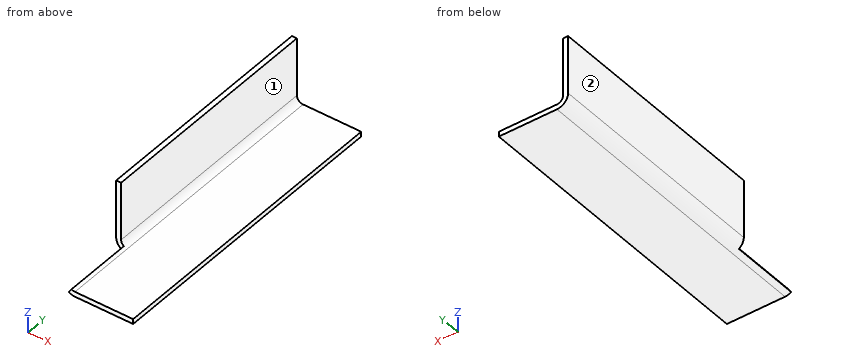
from build123d import *

# Parameters (mm, degrees)
SKETCH1_W                    = 28
SKETCH1_H                    = 122
BASE_FLANGE1_DEPTH           = 2
EDGE_FLANGE1_STRIP_W         = 13
EDGE_FLANGE1_STRIP_H         = 2
EDGE_FLANGE1_STRIP_CUT_DEPTH = 122
EDGE_FLANGE1_DEPTH           = 122
CUT_EXTRUDE1_START           = -61
CUT_EXTRUDE1_DEPTH           = 28


# Read off the part's stored shape, not the designer's step: Cut-Extrude1
# Sheet-metal steps are written as plain solids
with BuildPart() as part:
    # Sketch1 → Base-Flange1 (new body)
    with BuildSketch(Plane(origin=(0, 0, 0), x_dir=(0, 0, -1), z_dir=(1, 0, 0))):
        Rectangle(SKETCH1_W, SKETCH1_H)
    extrude(amount=-BASE_FLANGE1_DEPTH)

    # Edge-Flange1 strip (across the edge) → Edge-Flange1 strip cut (cut)
    with BuildSketch(Plane(origin=(0, -61, -14), x_dir=(0, 0, 1), z_dir=(0, 1, 0))):
        with Locations((-2, -1)):
            Rectangle(EDGE_FLANGE1_STRIP_W, EDGE_FLANGE1_STRIP_H)
    extrude(amount=EDGE_FLANGE1_STRIP_CUT_DEPTH, mode=Mode.SUBTRACT)

    # Edge-Flange1 section (across the edge) → Edge-Flange1 (add)
    with BuildSketch(Plane(origin=(0, -61, -14), x_dir=(0, 0, 1), z_dir=(0, 1, 0))):
        with BuildLine():
            Line((0, 2.5), (0, 26))
            Line((0, 26), (2, 26))
            Line((2, 26), (2, 2.5))
            ThreePointArc((2, 2.5), (2.732233047, 0.732233047), (4.5, 0))
            Line((4.5, 0), (4.5, -2))
            ThreePointArc((4.5, -2), (1.318019485, -0.681980515), (0, 2.5))
        make_face()
    extrude(amount=EDGE_FLANGE1_DEPTH)

    # Cut-Extrude1 outline → Cut-Extrude1 (cut)
    with BuildSketch(Plane(origin=(0, 0, 0), x_dir=(1, 0, 0), z_dir=(0, 1, 0)).offset(CUT_EXTRUDE1_START)):
        with BuildLine():
            Line((1.111111111, 11.578698548), (0, 13.241657386))
            ThreePointArc((0, 13.241657386), (-1.468626966, 11.621320343), (-2, 9.5))
            Line((-2, 9.5), (-2, -14))
            Line((-2, -14), (0, -14))
            Line((0, -14), (0, 9.5))
            ThreePointArc((0, 9.5), (0.295207241, 10.678511302), (1.111111111, 11.578698548))
        make_face()
    extrude(amount=CUT_EXTRUDE1_DEPTH, mode=Mode.SUBTRACT)


solid = part.part
Check sheet for the modelled part. Datum: model origin and axes. Units: mm. Face numbers are marked on the shaded views. A direction names the side the tool comes from. Give positions to 0.01 mm unless a question says otherwise; leave off trailing zeros. Write each loop counter-clockwise with the first axis right and the second up, starting at its lowest first coordinate (ties: lowest second). Pieces come first, ordered by that corner, then holes. Notation, with made-up numbers: (-15.75, -27) -> (39.25, -27) arc R23 cw to (39.25, -7) -> close; hole circle Ø8 at (-39, 32.5). An arc over 180 degrees is marked (long way). One line per item, written item: value. Start each with the question number.
Item 1: Material ranges on probe 1 along X at (y, z) = (29.5, 5.25); probe 2 along Z at (x, y) = (16.75, 52); probe 3 along Y at (x, z) = (-0.25, 3), recorded low to high. Write a range as from..to.
Item 2: Section check D-D on y = -47.5. Record the cut outline in (x, z).
Item 3: Tool access check on the marked faces 1 and 2. Record the directions out of +Z, -Z, +X, -X, +Y, -Y that give a thin tool (end or side, any length) a straight path to the whole face; none if there is none.
Item 4: Gauge pin test, flat ends, axial feed: pin 1 (1.6 mm diameter, centred on x = -0.5, z = -1, fed in from -Y); pin 2 (5 mm diameter, centred on x = 8.5, y = -1.5, fed in from +Z). Record the tip position at first contact, or that the pin passes through.
Item 5: Section check B-B on z = 1.5. Record the cut outline in (x, y), then the cut area to 3 significant figures.
Item 6: Section check C-C on x = 11.5. Record the cut outline in (y, z), then the cut area to 3 significant figures.
Item 7: Section check A-A on y = 47. Record the cut outline in (x, z).
Results list:
1. probe 1: -2..0
1. probe 2: -14..-12
1. probe 3: -33..61
2. outline: (0, -13.24) arc R4.5 ccw to (2.5, -14) -> (26, -14) -> (26, -12) -> (2.5, -12) arc R2.5 cw to (1.11, -11.58) -> close
3. face 1: +Z, +X, +Y, -Y
3. face 2: +Z, -Z, -X, +Y, -Y
4. pin 1: y = -33
4. pin 2: z = -12
5. outline: (-2, -33) -> (0, -33) -> (0, 61) -> (-2, 61) -> close
5. area: 188 mm²
6. outline: (-61, -14) -> (61, -14) -> (61, -12) -> (-61, -12) -> close
6. area: 244 mm²
7. outline: (-2, -9.5) arc R4.5 ccw to (2.5, -14) -> (26, -14) -> (26, -12) -> (2.5, -12) arc R2.5 cw to (0, -9.5) -> (0, 14) -> (-2, 14) -> close
